Verification items for the finished model (mm, model axes). Give positions to 0.01 mm unless a question says otherwise; leave off trailing zeros. Answer as a JSON object with one key per item and string values. Group by question number.
Item 1: Scan lines: line 1 along Z through (x, y) = (-17, -21); line 2 along X through (y, z) = (8, 16.5); line 3 along X through (y, z) = (-6, 13). Record each from-to range of solid material in increasing order. Write a range as [from, to].
Item 2: Go/stop test with a flat-tipped pin: pin 1 (3 mm diameter, centred on y = -12.5, z = 14.5, fed in from +X). Record where the tip stops, or that it passes through.
Item 3: Draft check along Z on faces 1 (the face through (-10, 0, 17.855)), 2 (the face through (-11, 25.4, 15)). Enter one of: +Z half, -Z half, draft (parallel to the pull), parting line (faces both ways), or undercut.
```python
from build123d import *

# Parameters (mm, degrees)
F1_DEPTH      = 25.4
F1_DEPTH_BACK = 25.4


with BuildPart() as f1:
    # F0 (on Front) → F1 (new body, two sides)
    with BuildSketch(Plane.XZ) as f1_sk:
        with BuildLine():
            Line((-10.3967804462, 17.8553387523), (-28.4781362861, 17.8553387523))
            add(Edge.make_bspline(
                [(-28.4781362861, 17.8553387523), (-26.151010961, 15.0979154646), (-21.8178408804, 9.6096851294), (-14.1950475719, 11.3771317015), (-11.8199229442, 6.8708596616), (-10.3967804462, 5.8764405549)],
                knots=[0, 0, 0, 0, 0.3899151773, 0.7013007932, 1, 1, 1, 1], degree=3))
            Line((-10.3967804462, 5.8764405549), (-10.3967804462, 17.8553387523))
        make_face()
        with BuildLine():
            Line((-10.3967804462, 17.8553387523), (-10.3967804462, 5.8764405549))
            add(Edge.make_bspline(
                [(7.6845753938, 17.8553387523), (5.3574500686, 15.0979154646), (1.0242799881, 9.6096851294), (-6.5985133204, 11.3771317015), (-8.9736379481, 6.8708596616), (-10.3967804462, 5.8764405549)],
                knots=[0, 0, 0, 0, 0.3899151773, 0.7013007932, 1, 1, 1, 1], degree=3))
            Line((7.6845753938, 17.8553387523), (-10.3967804462, 17.8553387523))
        make_face()
    extrude(amount=F1_DEPTH)
    extrude(f1_sk.sketch, amount=-F1_DEPTH_BACK)


solid = f1.part
```
Geometry check:
{
 "1": {"line 1": "[10.5, 17.86]", "line 2": "[-27.34, 6.54]", "line 3": "[-24.05, 3.26]"},
 "2": {"pin 1": "x = 6.12"},
 "3": {"face 1": "+Z half", "face 2": "draft"}
}
